Study the drawing (mm; zero at the part's minimum x, y, z) and answer. Round coordinates to 2 decimals unless told otherwise and drop trailing zeros. Write each loop counter-clockwise with the first axis right and the second up, starting at its lowest first coordinate (ties: lowest second). Pieces come first, ordered by that corner, then holes.
(1) A cutting plane is placed at B-B, the plane y = 1.2. Give the vertices of the cut face in (x, z).
(2) A cutting plane is placed at D-D, the plane z = 84. Give the vertices of the cut face in (x, y).
(3) A cutting plane is placed at C-C, the plane x = 40. Give the vertices of the cut face in (y, z), and give its area (3 significant figures).
(4) Find the intervals of material crossed by probe 1 along X at (y, z) = (1.45, 48); probe 2 along Z at (x, y) = (51.5, 0.85); probe 3 along X at (y, z) = (1.85, 55.5), in increasing order.
(5) Each of these flat-tipped pins is pushed along its axis until it touches: pin 1 Ø1 at (x, y) = (9.5, 1.5) entering from +Z; pin 2 Ø0.6 at (y, z) = (1, 83) entering from +X; pin 3 Ø15 at (x, z) = (40, 48) entering from +Y; pin 4 Ø1 at (y, z) = (1, 76) entering from -X. Where does it stop, or does it pass through?
(6) A cutting plane is placed at A-A, the plane z = 55.5. Give the vertices of the cut face in (x, y), and give its area (3 significant figures).
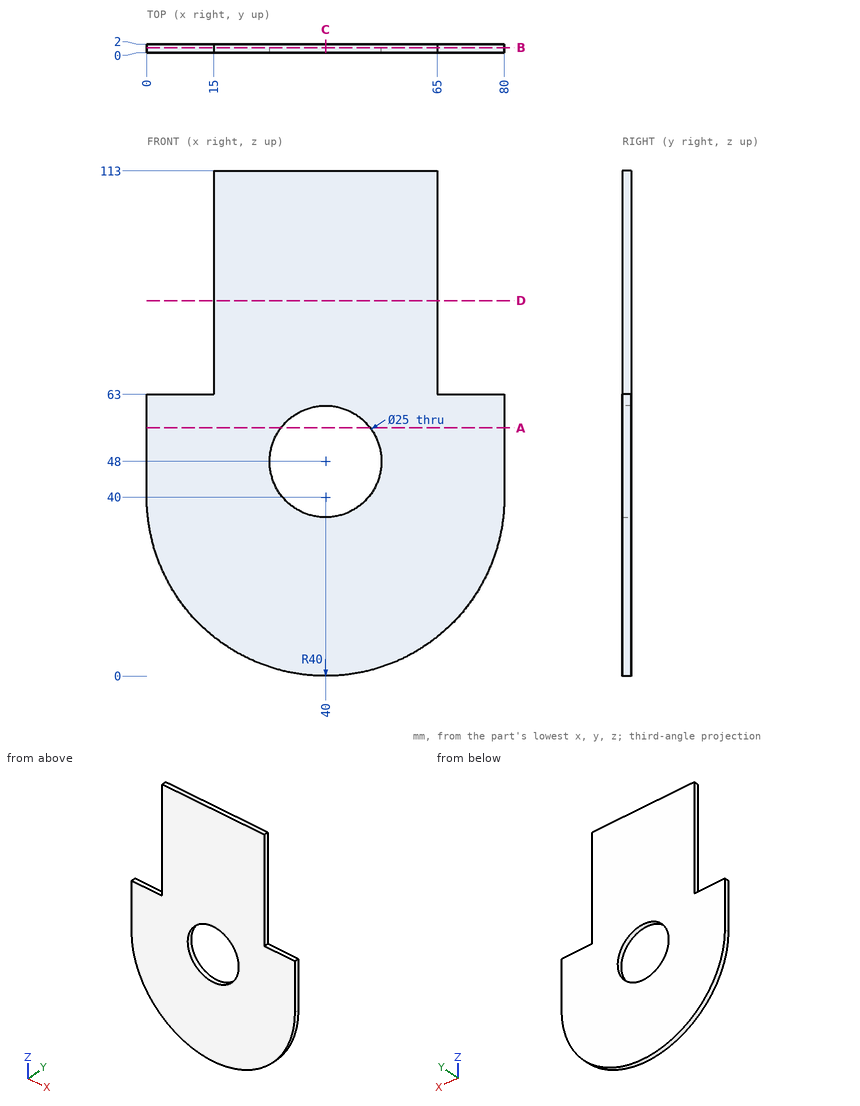
Solutions:
1. outline: (0, 40) arc R40 ccw to (80, 40) - (80, 63) - (65, 63) - (65, 113) - (15, 113) - (15, 63) - (0, 63) - close; hole circle Ø25 at (40, 48)
2. outline: (15, 0) - (65, 0) - (65, 2) - (15, 2) - close
3. outline: (0, 0) - (2, 0) - (2, 35.5) - (0, 35.5) - close; (0, 60.5) - (2, 60.5) - (2, 113) - (0, 113) - close
3. area: 176 mm2
4. probe 1: x = 0 to 27.5, 52.5 to 80
4. probe 2: z = 1.69 to 43.1, 52.9 to 113
4. probe 3: x = 0 to 30, 50 to 80
5. pin 1: stops at z = 63
5. pin 2: stops at x = 65
5. pin 3: passes through
5. pin 4: stops at x = 15
6. outline: (0, 0) - (30, 0) - (30, 2) - (0, 2) - close; (50, 0) - (80, 0) - (80, 2) - (50, 2) - close
6. area: 120 mm2
